Here's how the part is built. I have some questions about the finished solid (model axes, mm). A direction names the side the tool comes from. Round coordinates to 2 decimals unless told otherwise and drop trailing zeros. Order: outer loops, then holes, each group sorted by start corner. A loop starts at its lowest first (then second) coordinate and runs counter-clockwise, first axis right, second up. Notation, with made-up numbers: (-26.5, 7) -> (24.5, 7) arc R22 ccw to (24.5, 33) -> close; hole circle Ø2 at (-15, 20.25). An arc over 180 degrees is marked (long way). Use a Markdown table: item, result. Add a question column.
(1) I'm going to push flat-ended pins straight in: P1, Ø1.6, axis at x = 7, z = 10, coming from the +Y side; P2, Ø6, axis at x = 10, y = 11.5, coming from the +Z side; P3, Ø2.5, axis at x = 17.5, y = 0, coming from the +Z side; P4, Ø3, axis at y = -6.5, z = -4, coming from the +X side. Where does each tip first touch, or does it pass through?
(2) I want a section at B-B, the plane y = 12.5. Please give me the cut outline in (x, z), then the cut area to 3 significant figures.
(3) I want a section at A-A, the plane x = -3. Please give me the cut outline in (y, z).
(4) Thinking about a two-plate mould opening in Z: for faces 1 (the face through (11.958, 11.498, 0.198)), 2 (the face through (7, 0, -9)), 3 (the face through (0.6, -1.93, -9.99)), 4 (the face through (12, 9.1, -8.8)), which applies, pulls with the +Z half, pulls with the -Z half, needs draft (parallel to the pull), parting line crosses it, or undercut?
(5) On a 3-axis mill with a long thin cutter (end or side, diameter ignored), from which of +Z, -Z, +X, -X, +Y, -Y can I reach the whole of each face in a straight line? I mean faces 5 (the face through (12, -7.2, -0.1)), 6 (the face through (3, -2.5, -10)), 7 (the face through (7, 0, 9)), 8 (the face through (16, 1, 10)). Say none if no direction works.
(6) If I drill on probe 1 along X at (y, z) = (0, 10.25); probe 2 along Y at (x, z) = (17.5, -10.4); probe 3 along Z at (x, y) = (11, -3.25), over which ranges is the centre line in solid material (lowest first)?
(7) I want a section at C-C, the plane z = 6.5. Give the number of separate pieces and of enclosed holes in the cut face, then the cut area to 3 significant figures.
from build123d import *

# Parameters (mm, degrees)
SKETCH1_W                = 2
SKETCH1_H                = 5
BOSS_EXTRUDE1_DEPTH      = 15
BOSS_EXTRUDE1_2_DEPTH    = 15
SKETCH2_W                = 1
SKETCH2_H                = 5
BOSS_EXTRUDE2_DEPTH      = 5
CUT_EXTRUDE1_DEPTH       = 30.107559156
CUT_EXTRUDE1_DEPTH_BACK  = 30.107559156
SKETCH3_R                = 1.5
SWEEP1_START             = 9
SWEEP1_DEPTH             = 6
BOSS_EXTRUDE3_DEPTH      = 12
CUT_EXTRUDE2_DEPTH       = 5
FILLET1_R                = 2
BOSS_EXTRUDE6_START      = -6
SKETCH7_W                = 6
SKETCH7_H                = 2
BOSS_EXTRUDE6_DEPTH      = 46
BOSS_EXTRUDE7_DEPTH      = 3
BOSS_EXTRUDE7_DEPTH_BACK = 9
SKETCH8_R                = 1.5
FILLET2_R                = 2.5
BOSS_EXTRUDE10_DEPTH     = 15


# Read off the part's stored shape, not the designer's step: Sweep1
with BuildPart() as part:
    # Sketch1 → Boss-Extrude1 (new body)
    with BuildSketch(Plane(origin=(0, 0, 0), x_dir=(0, 0, -1), z_dir=(1, 0, 0))):
        with Locations((-10, 0)):
            Rectangle(SKETCH1_W, SKETCH1_H)
    extrude(amount=BOSS_EXTRUDE1_DEPTH)



with BuildPart() as body_2:
    # Sketch1 → Boss-Extrude1 2 (new body)
    with BuildSketch(Plane(origin=(0, 0, 0), x_dir=(0, 0, -1), z_dir=(1, 0, 0))):
        with Locations((10, 0)):
            Rectangle(SKETCH1_W, SKETCH1_H)
    extrude(amount=BOSS_EXTRUDE1_2_DEPTH)


with BuildPart() as part_1:
    add(part.part)

    add(body_2.part)  # Boss-Extrude2 merges body 2
    # Sketch2 → Boss-Extrude2 (add)
    with BuildSketch(Plane(origin=(15, 0, 0), x_dir=(0, 0, -1), z_dir=(1, 0, 0))):
        with Locations((10.5, 0)):
            Rectangle(SKETCH2_W, SKETCH2_H)
        with Locations((-10.5, 0)):
            Rectangle(SKETCH2_W, SKETCH2_H)
    extrude(amount=BOSS_EXTRUDE2_DEPTH)

    # Sketch3 → Cut-Extrude1 (cut, two sides: drawn at the far end of the back side and taken through both)
    with BuildSketch(Plane.XY.offset(-10).offset(-CUT_EXTRUDE1_DEPTH_BACK)):
        with Locations((17.5, 0)):
            Circle(SKETCH3_R)
    extrude(amount=CUT_EXTRUDE1_DEPTH + CUT_EXTRUDE1_DEPTH_BACK, mode=Mode.SUBTRACT)

    # Sweep1 outline → Sweep1 (add)
    with BuildSketch(Plane.YZ.offset(SWEEP1_START)):
        with BuildLine():
            ThreePointArc((2.5, -11), (13.5, 0), (2.5, 11))
            Line((2.5, 11), (2.5, 9))
            ThreePointArc((2.5, 9), (11.5, 0), (2.5, -9))
            Line((2.5, -9), (2.5, -11))
        make_face()
    extrude(amount=SWEEP1_DEPTH)

    # Sketch5 → Boss-Extrude3 (add)
    with BuildSketch(Plane(origin=(0, 0, 0), x_dir=(0, 0, -1), z_dir=(1, 0, 0))):
        with BuildLine():
            Line((-9, -2.5), (-11, -2.5))
            add(Edge.make_bspline(
                [(-11, -2.5), (-11, -8.980170496), (0, -8.980170496)],
                knots=[3.141592654, 3.141592654, 3.141592654, 4.71238898, 4.71238898, 4.71238898], degree=2, weights=[1, 0.707106781, 1]))
            Line((0, -8.980170496), (0, -7.009343108))
            add(Edge.make_bspline(
                [(-9, -2.5), (-9, -7.009343108), (0, -7.009343108)],
                knots=[3.141592654, 3.141592654, 3.141592654, 4.71238898, 4.71238898, 4.71238898], degree=2, weights=[1, 0.707106781, 1]))
        make_face()
    boss_extrude3 = extrude(amount=BOSS_EXTRUDE3_DEPTH)

    # Sketch6 → Cut-Extrude2 (cut)
    with BuildSketch(Plane.ZY):
        with BuildLine():
            Line((11, -2.5), (9, -2.5))
            add(Edge.make_bspline(
                [(0, -7.009343108), (9, -7.009343108), (9, -2.5)],
                knots=[4.71238898, 4.71238898, 4.71238898, 6.283185307, 6.283185307, 6.283185307], degree=2, weights=[1, 0.707106781, 1]))
            Line((0, -7.009343108), (0, -8.980170496))
            add(Edge.make_bspline(
                [(0, -8.980170496), (11, -8.980170496), (11, -2.5)],
                knots=[4.71238898, 4.71238898, 4.71238898, 6.283185307, 6.283185307, 6.283185307], degree=2, weights=[1, 0.707106781, 1]))
        make_face()
    cut_extrude2 = extrude(amount=-CUT_EXTRUDE2_DEPTH, mode=Mode.SUBTRACT)

    # Mirror2: Boss-Extrude3, Cut-Extrude2 across plane
    add(boss_extrude3.mirror(Plane(origin=(12, -8.980170496, 0), x_dir=(1, 0, 0), z_dir=(0, 0, 1))))
    add(cut_extrude2.mirror(Plane(origin=(12, -8.980170496, 0), x_dir=(1, 0, 0), z_dir=(0, 0, 1))), mode=Mode.SUBTRACT)

    # Fillet1
    fillet1_edges = [part_1.edges().sort_by_distance(p)[0] for p in [
        (0, -2.5, -10),
        (0, 2.5, -10),
        (0, 2.5, 10),
        (0, -2.5, 10),
    ]]
    fillet(fillet1_edges, radius=FILLET1_R)

    # Sketch7 → Boss-Extrude6 (add)
    with BuildSketch(Plane.ZY.offset(-9).offset(BOSS_EXTRUDE6_START)):
        with Locations((0, 12.5)):
            Rectangle(SKETCH7_W, SKETCH7_H)
    extrude(amount=BOSS_EXTRUDE6_DEPTH)

    # Sketch8 → Boss-Extrude7 (add, two sides: drawn at the far end of the back side and taken through both)
    with BuildSketch(Plane.XY.offset(3).offset(-BOSS_EXTRUDE7_DEPTH_BACK)):
        with Locations((-31, 12.5)):
            Circle(SKETCH8_R)
    extrude(amount=BOSS_EXTRUDE7_DEPTH + BOSS_EXTRUDE7_DEPTH_BACK)

    # Fillet2
    fillet2_edges = [part_1.edges().sort_by_distance(p)[0] for p in [
        (20, -2.5, -10.5),
        (20, -2.5, 10.5),
    ]]
    fillet(fillet2_edges, radius=FILLET2_R)

    # 3DSketch3 → Boss-Extrude10 (add)
    with BuildSketch(Plane(origin=(-15, 7.995255445, 9.529017137), x_dir=(0, 0, -1), z_dir=(1, 0, 0))):
        with BuildLine():
            Line((0, 0), (2, 0))
            ThreePointArc((2, 0), (9.529017137, 3.825899604), (17.058034273, 0))
            Line((17.058034273, 0), (19.058034273, 0))
            ThreePointArc((19.058034273, 0), (15.031388903, 4.029654263), (9.529017137, 5.504744555))
            ThreePointArc((9.529017137, 5.504744555), (4.026645371, 4.029654263), (0, 0))
        make_face()
    extrude(amount=BOSS_EXTRUDE10_DEPTH)


solid = part_1.part
Taken from the geometry:
| question | item | result |
|---|---|---|
| 1 | P1 | stops at y = 2.5 |
| 1 | P2 | stops at z = 9.22 |
| 1 | P3 | passes through |
| 1 | P4 | stops at x = 12 |
| 2 | outline | (-32.5, -6) -> (-29.5, -6) -> (-29.5, -3) -> (-15, -3) -> (-15, -4.58) -> (0, -4.58) -> (0, -3) -> (9, -3) -> (9, -4.58) -> (15, -4.58) -> (15, 4.58) -> (9, 4.58) -> (9, 3) -> (0, 3) -> (0, 4.58) -> (-15, 4.58) -> (-15, 3) -> (-29.5, 3) -> (-29.5, 6) -> (-32.5, 6) -> close |
| 2 | area | 369 mm2 |
| 3 | outline | (8, -9.53) arc R11 ccw to (13.08, -3) -> (13.5, -3) -> (13.5, 3) -> (13.08, 3) arc R11 ccw to (8, 9.53) -> (8, 7.53) arc R9.32 cw to (11.5, 2.43) -> (11.5, -2.43) arc R9.32 cw to (8, -7.53) -> close |
| 4 | face 1 | undercut |
| 4 | face 2 | undercut |
| 4 | face 3 | needs draft |
| 4 | face 4 | pulls with the -Z half |
| 5 | face 5 | +Z, -Z, +X, -Y |
| 5 | face 6 | +Z, -Z, -X, -Y |
| 5 | face 7 | +X, -X |
| 5 | face 8 | +X, +Y, -Y |
| 6 | probe 1 | x = 0 to 16, 19 to 20 |
| 6 | probe 2 | y = -2.5 to -1.5, 1.5 to 2.5 |
| 6 | probe 3 | z = -10.93 to -8.87, 8.87 to 10.93 |
| 7 | separate pieces | 3 |
| 7 | enclosed holes | 0 |
| 7 | area | 63.6 mm2 |
